```python
from build123d import *

# Parameters (mm, degrees)
F1_DEPTH      = 10
F2_W          = 22
F2_H          = 5
F3_DEPTH      = 40
F4_W          = 1.8184431829
F4_H          = 3.4095803276
F4_R          = 1.65
F5_DEPTH      = 25
F5_DEPTH_BACK = 25
F7_DEPTH      = 50.001


with BuildPart() as f1:
    # F0 (on Top) → F1 (new body)
    with BuildSketch(Plane.XY):
        Polygon((0, 15), (0, 0), (6, 0), (6, 10), (16, 10), (16, 0), (22, 0), (22, 15), align=None)
    extrude(amount=F1_DEPTH)

    # F2 (on face) → F3 (join)
    with BuildSketch(Plane.XY.offset(10)):
        with Locations((11, 12.5)):
            Rectangle(F2_W, F2_H)
    extrude(amount=F3_DEPTH)

    # F4 (on face) → F5 (cut, two sides)
    with BuildSketch(Plane.XZ.offset(-10)) as f5_sk:
        with Locations((3.9092215914, 14.5157719962)):
            Rectangle(F4_W, F4_H)
        with Locations((18.0907784086, 14.5157719962)):
            Rectangle(F4_W, F4_H)
        with Locations((18.5, 2.5)):
            Circle(F4_R)
        with Locations((3.5, 2.5)):
            Circle(F4_R)
        with Locations((18.0907784086, 29.5157719962)):
            Rectangle(F4_W, F4_H)
        with Locations((18.0907784086, 44.5157719962)):
            Rectangle(F4_W, F4_H)
        with Locations((3.9092215914, 29.5157719962)):
            Rectangle(F4_W, F4_H)
        with Locations((3.9092215914, 44.5157719962)):
            Rectangle(F4_W, F4_H)
        with Locations((18.5, 7.5)):
            Circle(F4_R)
        with Locations((3.5, 7.5)):
            Circle(F4_R)
    extrude(amount=-F5_DEPTH, mode=Mode.SUBTRACT)
    extrude(f5_sk.sketch, amount=F5_DEPTH_BACK, mode=Mode.SUBTRACT)

    # F6 (on face) → F7 (cut, through all)
    with BuildSketch(Plane.XY.offset(50)):
        with BuildLine():
            Line((6, 10), (16, 10))
            ThreePointArc((16, 10), (11, 11.2785394519), (6, 10))
        make_face()
    extrude(amount=-F7_DEPTH, mode=Mode.SUBTRACT)


solid = f1.part
```
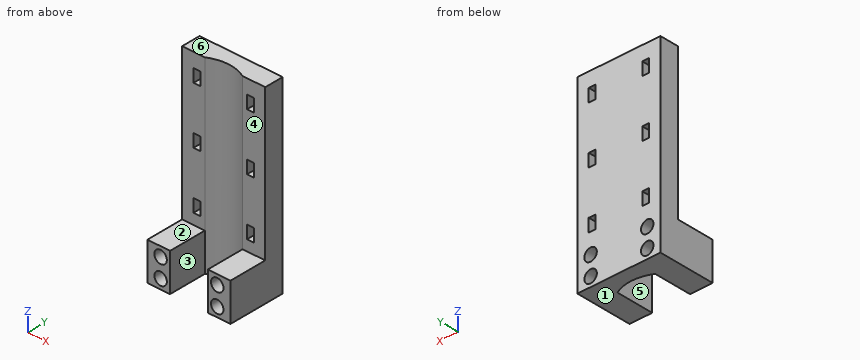
CAD build for the part. Positions are in the model's coordinates, mm. Face numbers are marked on the shaded views. A direction names the side the tool comes from. Coordinates: 2 decimals unless noted, no trailing zeros. Write each loop counter-clockwise with the first axis right and the second up, starting at its lowest first coordinate (ties: lowest second). Pieces come first, ordered by that corner, then holes. Notation, with made-up numbers: (37.5, 36) -> (95.5, 36) arc R16 cw to (95.5, 40) -> close; hole circle Ø6 at (9.5, 24). An arc over 180 degrees is marked (long way). Return JSON: item names as keys, results as strings. Group by question number.
Q1. Cut at D-D, the plane z = 18. Give the cut face in (x, y), then the cut area to 3 significant figures.
Q2. Cut at C-C, the plane z = 2.5. Give the cut face in (x, y).
Q3. Which spindle directions (+Z, -Z, +X, -X, +Y, -Y) get a long thin tool onto all of the face, cutting with end or side? Do the marked faces 4, 5 and 6. Say none if no direction does.
Q4. Cut at A-A, the plane y = 1.5. Give the cut face in (x, z).
Q5. Pull direction Z, two halves, no side cores. Call the marked faces 1, 2 and 3: released by +Z, released by -Z, zero draft, split by the parting line, or undercut.
Q6. Cut at B-B, the plane x = 3.5. Give the cut face in (y, z).
Q7. Flat gauge pins, fed straight in: pin 1 (2 mm diameter, centred on x = 3.5, z = 7.5, fed in from +Y); pin 2 (5 mm diameter, centred on x = 1.5, z = 20, fed in from -Y). Where does each tip first touch, or does it go through?
Q8. Drill centre lines: line 1 (Z direction, x = 18.5, y = 6.75); line 2 (X direction, y = 6, z = 2.5); line 3 (X direction, y = 9, z = 3.5). Where is each one in solid material? Low to high.
Returned:
{
 "1": {"outline": "(0, 10) -> (6, 10) arc R10.42 cw to (16, 10) -> (22, 10) -> (22, 15) -> (0, 15) -> close", "area": "101 mm2"},
 "2": {"outline": "(0, 0) -> (1.85, 0) -> (1.85, 15) -> (0, 15) -> close; (5.15, 0) -> (6, 0) -> (6, 10) arc R10.42 cw to (16, 10) -> (16, 0) -> (16.85, 0) -> (16.85, 15) -> (5.15, 15) -> close; (20.15, 0) -> (22, 0) -> (22, 15) -> (20.15, 15) -> close"},
 "3": {"face 4": "+Z, +X, -X, -Y", "face 5": "+Z, -Z, -Y", "face 6": "+Z, +X, -X, +Y, -Y"},
 "4": {"outline": "(0, 0) -> (6, 0) -> (6, 10) -> (0, 10) -> close; (16, 0) -> (22, 0) -> (22, 10) -> (16, 10) -> close; hole circle Ø3.3 at (3.5, 2.5); hole circle Ø3.3 at (3.5, 7.5); hole circle Ø3.3 at (18.5, 2.5); hole circle Ø3.3 at (18.5, 7.5)"},
 "5": {"face 1": "released by -Z", "face 2": "released by +Z", "face 3": "zero draft"},
 "6": {"outline": "(0, 0) -> (15, 0) -> (15, 0.85) -> (0, 0.85) -> close; (0, 4.15) -> (15, 4.15) -> (15, 5.85) -> (0, 5.85) -> close; (0, 9.15) -> (15, 9.15) -> (15, 12.81) -> (10, 12.81) -> (10, 10) -> (0, 10) -> close; (10, 16.22) -> (15, 16.22) -> (15, 27.81) -> (10, 27.81) -> close; (10, 31.22) -> (15, 31.22) -> (15, 42.81) -> (10, 42.81) -> close; (10, 46.22) -> (15, 46.22) -> (15, 50) -> (10, 50) -> close"},
 "7": {"pin 1": "passes through", "pin 2": "stops at y = 10"},
 "8": {"line 1": "z = 0 to 0.85, 4.15 to 5.85, 9.15 to 10", "line 2": "x = 0 to 1.85, 5.15 to 6, 16 to 16.85, 20.15 to 22", "line 3": "x = 0 to 2.19, 4.81 to 6, 16 to 17.19, 19.81 to 22"}
}
